Check sheet for the drawn part. Datum: minimum x, y, z corner. Units: mm. Give positions to 0.01 mm unless a question says otherwise; leave off trailing zeros. Write each loop counter-clockwise with the first axis right and the second up, starting at its lowest first coordinate (ties: lowest second). Pieces come first, ordered by that corner, then holes. Notation, with made-up numbers: M 37.25,12 L 78.25,12 A15 cw 78.25,37 Z; hole C 45.25,12.25 d3. An arc over 180 degrees is marked long. Write item = value, one per line. Start each with the question number.
1) Gauge pin test, flat end, axial feed: pin 1 (1 mm diameter, centred on x = 45.73, y = 38.45, fed in from +Z). Record the tip position at first contact, or that the pin passes through.
2) Sectioned sample at A-A, the plane y = 2. Record the cut outline in (x, z).
3) Sectioned sample at D-D, the plane y = 27. Record the cut outline in (x, z) (1 decimal).
4) Scan lines: L1, parallel to X at y = 38.45, z = 0.8; L2, parallel to X at y = 30, z = 0.4; L3, parallel to X at y = 19, z = 0.4 (1 decimal). Record each from-to range of solid material in increasing order.
5) Sectioned sample at C-C, the plane x = 13. Record the cut outline in (y, z).
6) Sectioned sample at B-B, the plane z = 0.75. Count the separate pieces of the cut face and the enclosed holes in it, then the cut area to 3 significant figures.
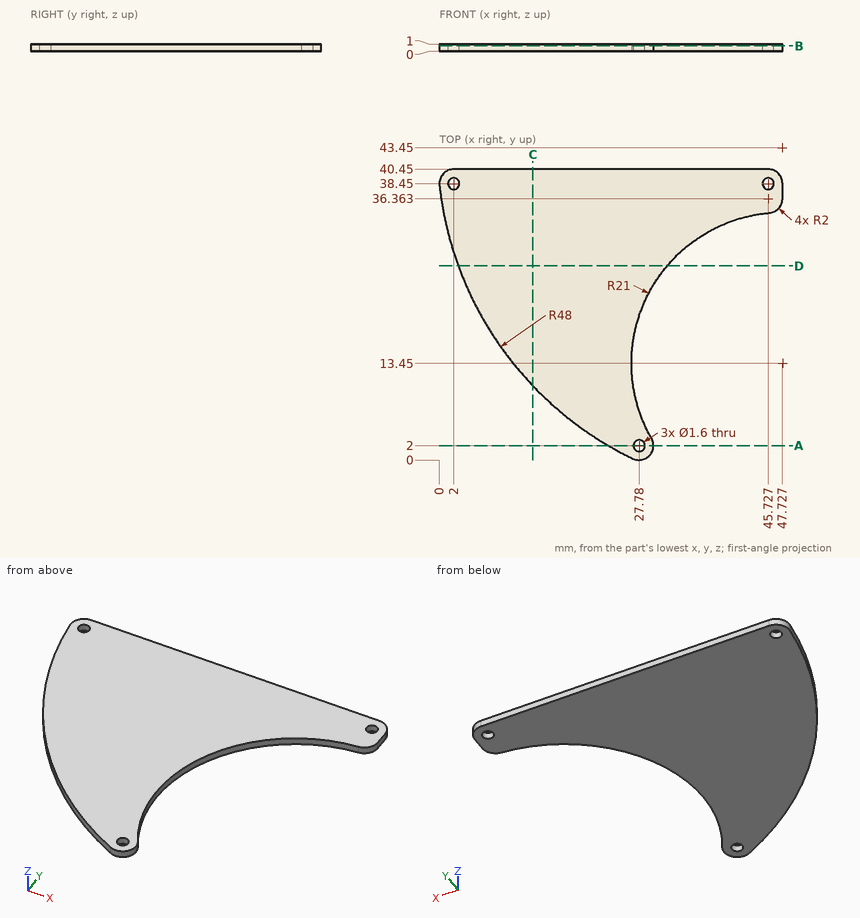
Data:
q1.pin_1 = through
q2.outline = M 23.52,0 L 26.98,0 L 26.98,1 L 23.52,1 Z; M 28.58,0 L 29.78,0 L 29.78,1 L 28.58,1 Z
q3.outline = M 2.6,0 L 31.7,0 L 31.7,1 L 2.6,1 Z
q4.L1 = 0 to 1.2, 2.8 to 44.93, 46.53 to 47.73
q4.L2 = 1.65 to 34.8
q4.L3 = 6.4 to 27.5
q5.outline = M 10.31,0 L 40.45,0 L 40.45,1 L 10.31,1 Z
q6.separate_pieces = 1
q6.enclosed_holes = 3
q6.area = 983 mm2
